Could you check a few things on this model? Use its own coordinates, in mm. A direction names the side the tool comes from. Round coordinates to 2 decimals unless told otherwise and drop trailing zeros. Loops run counter-clockwise (first coordinate to the right, second up) from the corner with the lowest first, then second, coordinate; pieces in that order, holes last.
from build123d import *

# Parameters (mm, degrees)
SKETCH_1_R           = 4.5
SKETCH_1_R_2         = 2.057142857
EXTRUDE_1_DEPTH      = 15
SKETCH_2_OUTSIDE_W   = 15.842
SKETCH_2_OUTSIDE_H   = 15.842
SKETCH_2_OUTSIDE_R   = 3
CUT_EXTRUDE_1_DEPTH  = 13
CUT_EXTRUDE_1_DRAFT  = 2
SKETCH_3_OUTSIDE_W   = 14.934
SKETCH_3_OUTSIDE_H   = 14.934
SKETCH_3_OUTSIDE_W_2 = 5
SKETCH_3_OUTSIDE_H_2 = 5
CUT_EXTRUDE_2_DEPTH  = 8
FILLET_2_R           = 0.5
FILLET_3_R           = 0.5
FILLET_4_R           = 0.5
FILLET_5_R           = 0.5


with BuildPart() as part:
    # Эскиз1 → Бобышка-Вытянуть1 (new body)
    with BuildSketch(Plane.XY):
        Circle(SKETCH_1_R)
        Circle(SKETCH_1_R_2, mode=Mode.SUBTRACT)
    extrude(amount=EXTRUDE_1_DEPTH)


with BuildPart() as cut_extrude_1_tool:
    # Эскиз2 outside → Вырез-Вытянуть1 (with draft: the straight prism first)
    with BuildSketch(Plane.XY.offset(15)):
        Rectangle(SKETCH_2_OUTSIDE_W, SKETCH_2_OUTSIDE_H)
        Circle(SKETCH_2_OUTSIDE_R, mode=Mode.SUBTRACT)
    extrude(amount=-CUT_EXTRUDE_1_DEPTH)
    # Вырез-Вытянуть1: the draft: its side faces are tilted about the plane it starts from
    cut_extrude_1_sides = [cut_extrude_1_tool.faces().sort_by_distance(p)[0] for p in [
        (0, -7.921, 8.5),
        (7.921, 0, 8.5),
        (0, 7.921, 8.5),
        (-7.921, 0, 8.5),
        (-3, 0, 8.5),
    ]]
    draft(cut_extrude_1_sides, Plane.XY.offset(15), CUT_EXTRUDE_1_DRAFT)


with BuildPart() as part_1:
    add(part.part)

    # Вырез-Вытянуть1: cut by cut_extrude_1_tool
    add(cut_extrude_1_tool.part, mode=Mode.SUBTRACT)

    # Эскиз3 outside → Вырез-Вытянуть2 (cut)
    with BuildSketch(Plane.XY.offset(15)):
        Rectangle(SKETCH_3_OUTSIDE_W, SKETCH_3_OUTSIDE_H)
        Rectangle(SKETCH_3_OUTSIDE_W_2, SKETCH_3_OUTSIDE_H_2, mode=Mode.SUBTRACT)
    extrude(amount=-CUT_EXTRUDE_2_DEPTH, mode=Mode.SUBTRACT)

    # Скругление2
    # the kernel refuses this fillet: 0.5 mm, written as the material it takes off along each edge
    with BuildSketch(Plane(origin=(0, 0, 15), x_dir=(0.9881342002725989, 0.15359297591892496, 0), z_dir=(0.15359297591892496, -0.9881342002725989, 0))) as fillet_2_piece_1:
        with BuildLine():
            CenterArc((3 - FILLET_2_R * 1.03553031379, -FILLET_2_R), FILLET_2_R, 358, 92)
            Line((3 - FILLET_2_R * 1.03553031379, 0), (3, 0))
            Line((3, 0), (3 - FILLET_2_R * 0.0361394867715, -FILLET_2_R * 1.0348994967))
        make_face()
    revolve(axis=Axis((0, 0, 15), (0, 0, 1)), revolution_arc=72.329594827, mode=Mode.SUBTRACT)
    with BuildSketch(Plane(origin=(0, 0, 15), x_dir=(-0.1535929759189553, 0.9881342002725941, 0), z_dir=(0.9881342002725941, 0.1535929759189553, 0))) as fillet_2_piece_2:
        with BuildLine():
            CenterArc((3 - FILLET_2_R * 1.03553031379, -FILLET_2_R), FILLET_2_R, 358, 92)
            Line((3 - FILLET_2_R * 1.03553031379, 0), (3, 0))
            Line((3, 0), (3 - FILLET_2_R * 0.0361394867715, -FILLET_2_R * 1.0348994967))
        make_face()
    revolve(axis=Axis((0, 0, 15), (0, 0, 1)), revolution_arc=72.329594827, mode=Mode.SUBTRACT)
    with BuildSketch(Plane(origin=(0, 0, 15), x_dir=(-0.9881342002725968, -0.15359297591893833, 0), z_dir=(-0.15359297591893833, 0.9881342002725968, 0))) as fillet_2_piece_3:
        with BuildLine():
            CenterArc((3 - FILLET_2_R * 1.03553031379, -FILLET_2_R), FILLET_2_R, 358, 92)
            Line((3 - FILLET_2_R * 1.03553031379, 0), (3, 0))
            Line((3, 0), (3 - FILLET_2_R * 0.0361394867715, -FILLET_2_R * 1.0348994967))
        make_face()
    revolve(axis=Axis((0, 0, 15), (0, 0, 1)), revolution_arc=72.329594827, mode=Mode.SUBTRACT)
    with BuildSketch(Plane(origin=(0, 0, 15), x_dir=(0.15359297591892515, -0.9881342002725989, 0), z_dir=(-0.9881342002725989, -0.15359297591892515, 0))) as fillet_2_piece_4:
        with BuildLine():
            CenterArc((3 - FILLET_2_R * 1.03553031379, -FILLET_2_R), FILLET_2_R, 358, 92)
            Line((3 - FILLET_2_R * 1.03553031379, 0), (3, 0))
            Line((3, 0), (3 - FILLET_2_R * 0.0361394867715, -FILLET_2_R * 1.0348994967))
        make_face()
    revolve(axis=Axis((0, 0, 15), (0, 0, 1)), revolution_arc=72.329594827, mode=Mode.SUBTRACT)
    with BuildSketch(Plane(origin=(2.5, 2.908312395, 15), x_dir=(-1, 0, 0), z_dir=(0, -1, 0)), Plane(origin=(2.908312395, -2.5, 15), x_dir=(0, 1, 0), z_dir=(-1, 0, 0)), Plane(origin=(-2.5, -2.908312395, 15), x_dir=(1, 0, 0), z_dir=(0, 1, 0)), Plane(origin=(-2.908312395, 2.5, 15), x_dir=(0, -1, 0), z_dir=(1, 0, 0))) as fillet_2_piece_5:
        with BuildLine():
            CenterArc((FILLET_2_R, FILLET_2_R), FILLET_2_R, 180, 90)
            Line((0, FILLET_2_R), (0, 0))
            Line((0, 0), (FILLET_2_R, 0))
        make_face()
    extrude(amount=5.81662479, mode=Mode.SUBTRACT)

    # Скругление3
    fillet_3_edges = [part_1.edges().sort_by_distance(p)[0] for p in [
        (-2.546029997, 0, 2),
    ]]
    fillet(fillet_3_edges, radius=FILLET_3_R)

    # Скругление4
    fillet_4_edges = [part_1.edges().sort_by_distance(p)[0] for p in [
        (-4.5, 0, 2),
    ]]
    fillet(fillet_4_edges, radius=FILLET_4_R)

    # Скругление5
    fillet_5_edges = [part_1.edges().sort_by_distance(p)[0] for p in [
        (-4.5, 0, 0),
    ]]
    fillet(fillet_5_edges, radius=FILLET_5_R)


solid = part_1.part
Item 1: If we section it at C-C, the plane z = 12.5: Please give me the cut outline in (x, y).
Results list:
outline: (-2.5, -1.49) arc R2.91 ccw to (-1.49, -2.5) - (1.49, -2.5) arc R2.91 ccw to (2.5, -1.49) - (2.5, 1.49) arc R2.91 ccw to (1.49, 2.5) - (-1.49, 2.5) arc R2.91 ccw to (-2.5, 1.49) - close; hole circle Ø4.11 at (0, 0)
Item 2: We'd pull the mould along X, two halves only. Please class faces 1 (the conical face through (-2.012, 1.845, 7.254)), 2 (the cylindrical face through (1.96, 0.62, 7.4)), 3 (the flat face through (2.5, 0, 11)), 4 (the flat face through (1.6, 1.6, 15)): released by +X, released by -X, zero draft, split by the parting line, or undercut.
Results list:
face 1: split by the parting line
face 2: undercut
face 3: released by +X
face 4: zero draft
Item 3: If I drill on line 1 along X through (y, z) = (0, 10.25); line 2 along X through (y, z) = (0, 5.25); line 3 along Y through (x, z) = (0, 4.5), over which ranges is the centre line in solid material (lowest first)?
Results list:
line 1: x = -2.5 to -2.06, 2.06 to 2.5
line 2: x = -2.66 to -2.06, 2.06 to 2.66
line 3: y = -2.63 to -2.06, 2.06 to 2.63
Item 4: Will these pins go through, and if not, where does the flat tip stop? pin 1 (3.5 mm diameter, centred on x = 0, z = 10, fed in from -Y); pin 2 (1.5 mm diameter, centred on y = -3.5, z = 9.5, fed in from +X); pin 3 (3.5 mm diameter, centred on y = 0, z = 11.5, fed in from +X); pin 4 (1 mm diameter, centred on y = -2, z = 8.5, fed in from +X).
Results list:
pin 1: stops at y = -2.5
pin 2: passes through
pin 3: stops at x = 2.5
pin 4: stops at x = 2.33
Item 5: If we section it at A-A, the plane x = 0: Please give me the cut outline in (y, z), then the cut area to 3 significant figures.
Results list:
outline: (-4.5, 0.5) arc R0.5 ccw to (-4, 0) - (-2.06, 0) - (-2.06, 15) arc R0.5 ccw to (-2.5, 14.5) - (-2.5, 7) - (-2.72, 7) - (-2.56, 2.52) arc R0.5 cw to (-3.06, 2) - (-4, 2) arc R0.5 ccw to (-4.5, 1.5) - close; (2.06, 0) - (4, 0) arc R0.5 ccw to (4.5, 0.5) - (4.5, 1.5) arc R0.5 ccw to (4, 2) - (3.06, 2) arc R0.5 cw to (2.56, 2.52) - (2.72, 7) - (2.5, 7) - (2.5, 14.5) arc R0.5 ccw to (2.06, 15) - close
area: 22.4 mm2
Item 6: If we section it at D-D, the plane z = 14.25: Please give me the cut outline in (x, y).
Results list:
outline: (-2.5, -1.61) arc R2.97 ccw to (-1.61, -2.5) - (1.61, -2.5) arc R2.97 ccw to (2.5, -1.61) - (2.5, 1.61) arc R2.97 ccw to (1.61, 2.5) - (-1.61, 2.5) arc R2.97 ccw to (-2.5, 1.61) - close; hole circle Ø4.11 at (0, 0)
Item 7: For faces 5 (the flat face through (0, -2.5, 11)), 6 (the flat face through (0, 2.5, 11)), 7 (the flat face through (-2.5, 0, 11)), 8 (the flat face through (-1.6, -1.6, 15)), which set-ups out of +Z, -Z, +X, -X, +Y, -Y let a thin tool reach every point of the face, with its end or its side?
Results list:
face 5: +Z, +X, -X, -Y
face 6: +Z, +X, -X, +Y
face 7: +Z, -X, +Y, -Y
face 8: +Z, +X, -X, +Y, -Y
